```python
from build123d import *

# Parameters (mm, degrees)
SKETCH1_W           = 90
SKETCH1_H           = 10
BOSS_EXTRUDE1_DEPTH = 25
BOSS_EXTRUDE2_START = 9
SKETCH1_3_R         = 20
SKETCH1_3_R_2       = 10
BOSS_EXTRUDE2_DEPTH = 6
BOSS_EXTRUDE3_START = 15
SKETCH1_4_R         = 10
BOSS_EXTRUDE3_DEPTH = 15
SKETCH1_5_R         = 10
CUT_EXTRUDE1_DEPTH  = 47.5
SKETCH2_W           = 42
SKETCH2_H           = 15
CUT_EXTRUDE2_DEPTH  = 110.658560997
BOSS_EXTRUDE4_START = -6
BOSS_EXTRUDE4_DEPTH = 18


with BuildPart() as part:
    # Sketch1 → Boss-Extrude1 (new, symmetric)
    with BuildSketch(Plane.XY):
        with Locations((0, -5)):
            Rectangle(SKETCH1_W, SKETCH1_H)
    extrude(amount=BOSS_EXTRUDE1_DEPTH, both=True)

    # Sketch1<3> → Boss-Extrude2 (add)
    # profile 1 of 3: a face of its own
    with BuildSketch(Plane.XY.offset(BOSS_EXTRUDE2_START)):
        Polygon((-25, 50), (25, 50), (45, 0), (-45, 0), align=None)
        with Locations((0, 35)):
            Circle(SKETCH1_3_R, mode=Mode.SUBTRACT)
    # profile 2 of 3: a face of its own
    with BuildSketch(Plane.XY.offset(BOSS_EXTRUDE2_START)):
        with BuildLine():
            Line((13.228756555, 50), (-13.228756555, 50))
            ThreePointArc((-13.228756555, 50), (-8.228756555, 16.771243445), (20, 35))
            ThreePointArc((20, 35), (18.228756555, 43.228756555), (13.228756555, 50))
        make_face()
        with Locations((0, 35)):
            Circle(SKETCH1_3_R_2, mode=Mode.SUBTRACT)
    # profile 3 of 3: a face of its own
    with BuildSketch(Plane.XY.offset(BOSS_EXTRUDE2_START)):
        with Locations((0, 35)):
            Circle(SKETCH1_3_R_2)
    boss_extrude2 = extrude(amount=BOSS_EXTRUDE2_DEPTH)

    # Mirror1: Boss-Extrude2 across plane
    add(boss_extrude2.mirror(Plane.XY))

    # Sketch1<4> → Boss-Extrude3 (add)
    # profile 1 of 2: a face of its own
    with BuildSketch(Plane.XY.offset(BOSS_EXTRUDE3_START)):
        with BuildLine():
            Line((13.228756555, 50), (-13.228756555, 50))
            ThreePointArc((-13.228756555, 50), (-8.228756555, 16.771243445), (20, 35))
            ThreePointArc((20, 35), (18.228756555, 43.228756555), (13.228756555, 50))
        make_face()
        with Locations((0, 35)):
            Circle(SKETCH1_4_R, mode=Mode.SUBTRACT)
    # profile 2 of 2: a face of its own
    with BuildSketch(Plane.XY.offset(BOSS_EXTRUDE3_START)):
        with BuildLine():
            ThreePointArc((13.228756555, 50), (0, 55), (-13.228756555, 50))
            Line((-13.228756555, 50), (13.228756555, 50))
        make_face()
    boss_extrude3 = extrude(amount=BOSS_EXTRUDE3_DEPTH)

    # Mirror2: Boss-Extrude3 across plane
    add(boss_extrude3.mirror(Plane.XY))

    # Sketch1<5> → Cut-Extrude1 (cut, symmetric)
    with BuildSketch(Plane.XY):
        with Locations((0, 35)):
            Circle(SKETCH1_5_R)
    extrude(amount=CUT_EXTRUDE1_DEPTH, both=True, mode=Mode.SUBTRACT)

    # Sketch2 → Cut-Extrude2 (cut, through all)
    with BuildSketch(Plane.ZY.offset(45)):
        with Locations((0, 57.5)):
            Rectangle(SKETCH2_W, SKETCH2_H)
    extrude(amount=-CUT_EXTRUDE2_DEPTH, mode=Mode.SUBTRACT)

    # Sketch3 → Boss-Extrude4 (add)
    with BuildSketch(Plane(origin=(0, 0, -15), x_dir=(-1, 0, 0), z_dir=(0, 0, -1)).offset(BOSS_EXTRUDE4_START)):
        Polygon((-45, 0), (-37, 20), (37, 20), (45, 0), align=None)
    extrude(amount=-BOSS_EXTRUDE4_DEPTH)


solid = part.part
```
Input: part model. Units: mm. Frame: model coordinates. A direction names the side the tool comes from. Coordinates: 2 decimals unless noted, no trailing zeros. Order: outer loops, then holes, each group sorted by start corner. A loop starts at its lowest first (then second) coordinate and runs counter-clockwise, first axis right, second up. Notation, with made-up numbers: (77, 19) - (134, 19) arc R28 ccw to (134, 38) - close; hole circle Ø4 at (72, 56.25). An arc over 180 degrees is marked (long way). Put each result on its own line as item: value.
1. Cut plane B-B on y = 31.5. Return the cut outline in (x, z), then the cut area to 3 significant figures.
Report:
outline: (-32.4, -15) - (-19.69, -15) - (-19.69, -30) - (-9.37, -30) - (-9.37, -9) - (-32.4, -9) - close; (-32.4, 9) - (-9.37, 9) - (-9.37, 30) - (-19.69, 30) - (-19.69, 15) - (-32.4, 15) - close; (9.37, -30) - (19.69, -30) - (19.69, -15) - (32.4, -15) - (32.4, -9) - (9.37, -9) - close; (9.37, 9) - (32.4, 9) - (32.4, 15) - (19.69, 15) - (19.69, 30) - (9.37, 30) - close
area: 1,170 mm2
2. Cut plane C-C on z = 3. Return the cut outline in (x, y).
Report:
outline: (-45, -10) - (45, -10) - (45, 0) - (37, 20) - (-37, 20) - (-45, 0) - close
3. Cut plane D-D on x = -17.5. Return the cut outline in (y, z), then the cut area to 3 significant figures.
Report:
outline: (-10, -25) - (0, -25) - (0, -15) - (25.32, -15) - (25.32, -30) - (44.68, -30) - (44.68, -15) - (50, -15) - (50, -9) - (20, -9) - (20, 9) - (50, 9) - (50, 15) - (44.68, 15) - (44.68, 30) - (25.32, 30) - (25.32, 15) - (0, 15) - (0, 25) - (-10, 25) - close
area: 2,040 mm2
4. Cut plane A-A on x = 0. Return the cut outline in (y, z).
Report:
outline: (-10, -25) - (0, -25) - (0, -15) - (15, -15) - (15, -30) - (25, -30) - (25, -9) - (20, -9) - (20, 9) - (25, 9) - (25, 30) - (15, 30) - (15, 15) - (0, 15) - (0, 25) - (-10, 25) - close; (45, -30) - (55, -30) - (55, -21) - (50, -21) - (50, -9) - (45, -9) - close; (45, 9) - (50, 9) - (50, 21) - (55, 21) - (55, 30) - (45, 30) - close
5. Contact query for flat-ended pins moving along their axis: pin 1 Ø6 at (x, y) = (26, 27.5) entering from -Z; pin 2 Ø5 at (x, z) = (-19.5, 20) entering from +Y; pin 3 Ø15 at (x, y) = (-5.5, 33.5) entering from -Z; pin 4 Ø6 at (x, y) = (32.5, 21) entering from +Z. Output: stop coordinate, or through.
Report:
pin 1: stops at z = -15
pin 2: stops at y = 45.54
pin 3: stops at z = -30
pin 4: stops at z = 15
6. Line query: line 1 along Y through (x, z) = (0, 19.5); line 2 along Z through (x, y) = (27, 41); line 3 along Z through (x, y) = (-15.5, 36). Output: solid intervals per line, ascending.
Report:
line 1: y = -10 to 0, 15 to 25, 45 to 50
line 2: z = -15 to -9, 9 to 15
line 3: z = -30 to -9, 9 to 30
7. Reachability of faces 1 (the face through (-1, -5, 25)), 2 (the face through (-1, 0, 20)), 3 (the face through (0, 52, 21)) from +Z, -Z, +X, -X, +Y, -Y: full face, straight path, thin tool, end or side. Return the list, or none.
Report:
face 1: +Z, +X, -X, -Y
face 2: +Z, +X, -X
face 3: +X, -X, +Y
8. Draft query along Z for faces 4 (the face through (-9, 40, -30)), 5 (the face through (1, 20, 0)), 6 (the face through (45, -5, 0)). Return one class per face: pulls with the +Z half, pulls with the -Z half, needs draft (parallel to the pull), parting line crosses it, or undercut.
Report:
face 4: pulls with the -Z half
face 5: undercut
face 6: needs draft
